Model file for the job. Use its own axes, mm. Round coordinates to 2 decimals unless told otherwise and drop trailing zeros. Loops run counter-clockwise (first coordinate to the right, second up) from the corner with the lowest first, then second, coordinate; pieces in that order, holes last. Notation, with made-up numbers: (-28.5, -31) -> (-12.5, -31) arc R23 ccw to (-12.5, -15) -> close; hole circle Ø8 at (-38.5, -38.5). An arc over 180 degrees is marked (long way). Use a Markdown table: item, result.
from build123d import *

# Parameters (mm, degrees)
BOSS_EXTRUDE1_DEPTH = 10


with BuildPart() as part:
    # Sketch1 → Boss-Extrude1 (new body)
    with BuildSketch(Plane.XY):
        with BuildLine():
            Line((0, 0), (35, 0))
            Line((35, 0), (55, -35))
            Line((55, -35), (55, -119))
            Line((55, -119), (13.21880537, -168.792888803))
            ThreePointArc((13.21880537, -168.792888803), (-12.876965195, -188.95866594), (-45, -196.425823621))
            ThreePointArc((-45, -196.425823621), (-83.079272466, -186.639009954), (-110.975129822, -158.932803869))
            Line((-110.975129822, -158.932803869), (-145, -100))
            Line((-145, -100), (-145, -20))
            Line((-145, -20), (-125, 0))
            Line((-125, 0), (-100, 0))
            ThreePointArc((-100, 0), (-89.393398282, -4.393398282), (-85, -15))
            Line((-85, -15), (-85, -30))
            Line((-85, -30), (-105, -30))
            ThreePointArc((-105, -30), (-112.071067812, -32.928932188), (-115, -40))
            Line((-115, -40), (-115, -85))
            ThreePointArc((-115, -85), (-106.213203436, -106.213203436), (-85, -115))
            Line((-85, -115), (-20, -115))
            ThreePointArc((-20, -115), (11.819805153, -101.819805153), (25, -70))
            Line((25, -70), (25, -30))
            Line((25, -30), (0, -30))
            ThreePointArc((0, -30), (-15, -15), (0, 0))
        make_face()
    extrude(amount=BOSS_EXTRUDE1_DEPTH)


solid = part.part
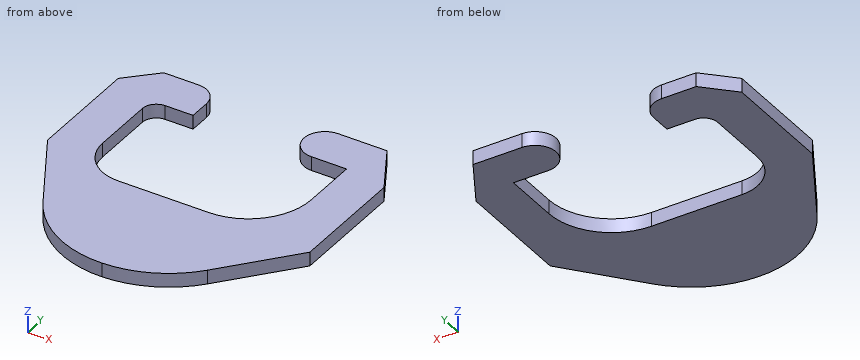
Q1. Band-saw the part on D-D, the plane x = -26. Give the cut face in (y, z).
Results list:
| item | result |
|---|---|
| outline | (-193.79, 0) -> (-115, 0) -> (-115, 10) -> (-193.79, 10) -> close |
Q2. Drill centre lines: L1, parallel to X at y = -70.5, z = 5.5; L2, parallel to X at y = -82.5, z = 5.5; L3, parallel to Y at x = 13, z = 5.75. Where is each one in solid material? Low to high. Write a range as from..to.
Results list:
| item | result |
|---|---|
| L1 | x = -145..-115, 25..55 |
| L2 | x = -145..-115, 23.23..55 |
| L3 | y = -169.05..-100.59, -30..0 |
Q3. Band-saw the part on C-C, the plane y = -12. Give the cut face in (x, z), plus the area to 3 significant figures.
Results list:
| item | result |
|---|---|
| outline | (-137, 0) -> (-85.3, 0) -> (-85.3, 10) -> (-137, 10) -> close; (-14.7, 0) -> (41.86, 0) -> (41.86, 10) -> (-14.7, 10) -> close |
| area | 1,080 mm² |
Q4. Band-saw the part on B-B, the plane z = 1.5. Give the cut face in (x, y).
Results list:
| item | result |
|---|---|
| outline | (-145, -100) -> (-110.98, -158.93) arc R75 ccw to (-45, -196.43) arc R77.38 ccw to (13.22, -168.79) -> (55, -119) -> (55, -35) -> (35, 0) -> (0, 0) arc R15 ccw to (0, -30) -> (25, -30) -> (25, -70) arc R45 cw to (-20, -115) -> (-85, -115) arc R30 cw to (-115, -85) -> (-115, -40) arc R10 cw to (-105, -30) -> (-85, -30) -> (-85, -15) arc R15 ccw to (-100, 0) -> (-125, 0) -> (-145, -20) -> close |
Q5. Flat gauge pins, fed straight in: pin 1 (3 mm diameter, centred on y = -21.5, z = 7.5, fed in from +X); pin 2 (6 mm diameter, centred on x = -74, z = 3, fed in from +Y); pin 3 (2 mm diameter, centred on x = -81, z = 7.5, fed in from -Y). Where does each tip first touch, or does it go through?
Results list:
| item | result |
|---|---|
| pin 1 | stops at x = 48.14 |
| pin 2 | stops at y = -115 |
| pin 3 | stops at y = -188.3 |
Q6. Band-saw the part on A-A, the plane y = -67. Give the cut face in (x, z), plus the area to 3 significant figures.
Results list:
| item | result |
|---|---|
| outline | (-145, 0) -> (-115, 0) -> (-115, 10) -> (-145, 10) -> close; (25, 0) -> (55, 0) -> (55, 10) -> (25, 10) -> close |
| area | 600 mm² |
